from build123d import *

# Parameters (mm, degrees)
F0_R     = 40
F1_DEPTH = 25
F2_R     = 12.5
F3_DEPTH = 25.001
F4_SIZE  = 1
F5_R     = 30
F5_R_2   = 25
F6_DEPTH = 15
F8_SIZE  = 0.5
F9_DEPTH = 10


# Not quite as in the source:
# - two fillets or chamfers of one size are made in one step


with BuildPart() as f1:
    # F0 (on Right) → F1 (new body)
    with BuildSketch(Plane.YZ):
        Circle(F0_R)
    extrude(amount=F1_DEPTH)

    # F2 (on face) → F3 (cut, through all)
    with BuildSketch(Plane(origin=(0, 0, 0), x_dir=(0, -1, 0), z_dir=(-1, 0, 0))):
        Circle(F2_R)
    extrude(amount=-F3_DEPTH, mode=Mode.SUBTRACT)

    # F4
    f4_edges = [f1.edges().sort_by_distance(p)[0] for p in [
        (0, -40, 0),
        (25, -40, 0),
    ]]
    chamfer(f4_edges, length=F4_SIZE)

    # F5 (on face) → F6 (cut)
    with BuildSketch(Plane.YZ.offset(25)):
        Circle(F5_R)
        Circle(F5_R_2, mode=Mode.SUBTRACT)
    extrude(amount=-F6_DEPTH, mode=Mode.SUBTRACT)

    # F8
    f8_edges = [f1.edges().sort_by_distance(p)[0] for p in [
        (25, -25, 0),
    ]]
    chamfer(f8_edges, length=F8_SIZE)

    # F5 (on face) → F9 (cut)
    with BuildSketch(Plane.YZ.offset(25)):
        Circle(F5_R)
        Circle(F5_R_2, mode=Mode.SUBTRACT)
    extrude(amount=-F9_DEPTH, mode=Mode.SUBTRACT)


solid = f1.part
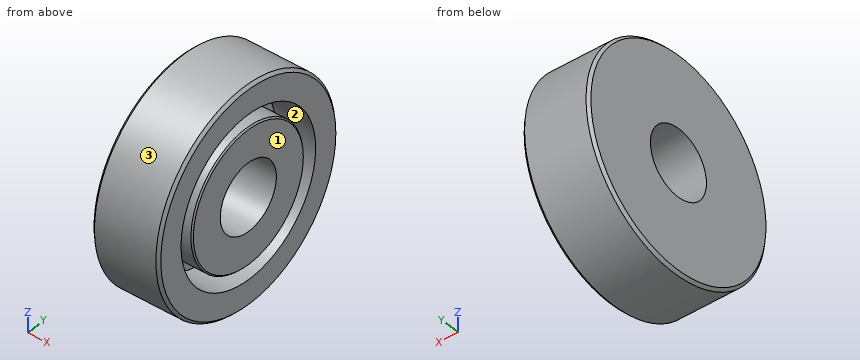
Model file for the job. Use its own axes, mm. Face numbers are marked on the shaded views. Coordinates: 2 decimals unless noted, no trailing zeros. Order: outer loops, then holes, each group sorted by start corner. A loop starts at its lowest first (then second) coordinate and runs counter-clockwise, first axis right, second up. Notation, with made-up numbers: (-11, 58) -> (2, 58) arc R17 ccw to (2, 76) -> close; hole circle Ø8 at (12, 80.5). An arc over 180 degrees is marked (long way). Return JSON: item names as keys, results as strings. Group by question number.
Item 1: Pull direction Z, two halves, no side cores. Call the marked faces 1, 2 and 3: pulls with the +Z half, pulls with the -Z half, needs draft (parallel to the pull), parting line crosses it, or undercut.
Item 2: Flat gauge pins, fed straight in: P1, Ø4, axis at x = 19.5, z = -24.5, coming from the -Y side; P2, Ø5, axis at x = 12, y = 19, coming from the +Z side; P3, Ø1, axis at x = 18.5, z = -1, coming from the +Y side. Where does each tip first touch, or does it go through?
Item 3: Saw through at A-A on z = 0. Write the cut outline in (x, y).
Item 4: Wall check: line 1 along Z through (x, y) = (9.75, 0); line 2 along Y through (x, z) = (11, 13.5); line 3 along X through (y, z) = (-1, 27). Give the ranges that are in metal, low to high. Write a range as [from, to].
Item 5: Saw through at C-C on x = 12.25. Write the cut outline in (y, z).
Item 6: Saw through at D-D on x = 2. Write the cut outline in (y, z).
Values found:
{
 "1": {"face 1": "needs draft", "face 2": "undercut", "face 3": "parting line crosses it"},
 "2": {"P1": "stops at y = -33.07", "P2": "stops at z = 36.44", "P3": "stops at y = 40"},
 "3": {"outline": "(0, -39) -> (1, -40) -> (24, -40) -> (25, -39) -> (25, -30) -> (10, -30) -> (10, -25) -> (24.5, -25) -> (25, -24.5) -> (25, -12.5) -> (0, -12.5) -> close; (0, 12.5) -> (25, 12.5) -> (25, 24.5) -> (24.5, 25) -> (10, 25) -> (10, 30) -> (25, 30) -> (25, 39) -> (24, 40) -> (1, 40) -> (0, 39) -> close"},
 "4": {"line 1": "z = [-40, -12.5], [12.5, 40]", "line 2": "y = [-37.65, -26.79], [-21.04, 21.04], [26.79, 37.65]", "line 3": "x = [0, 10]"},
 "5": {"outline": "circle Ø80 at (0, 0); circle Ø50 at (0, 0); hole circle Ø60 at (0, 0); hole circle Ø25 at (0, 0)"},
 "6": {"outline": "circle Ø80 at (0, 0); hole circle Ø25 at (0, 0)"}
}
